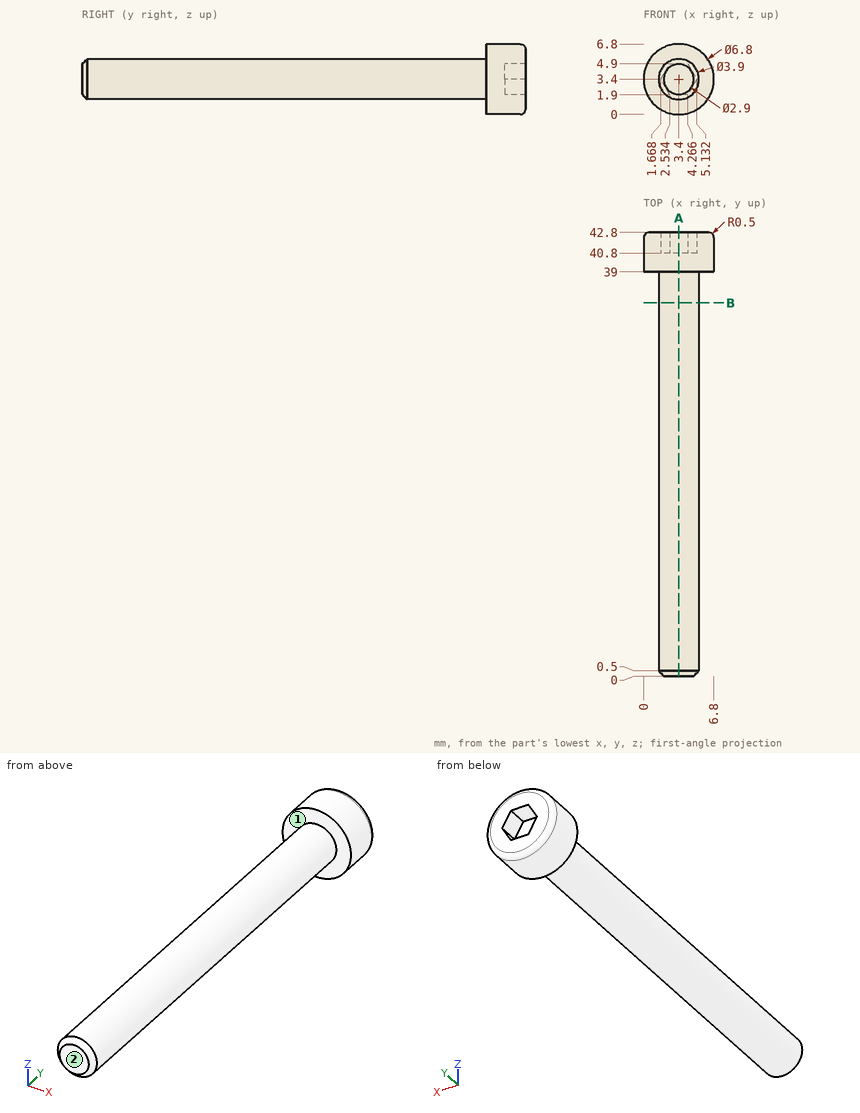
Print and shaded views of the part. All mm, measured from the part's lowest x, y and z. A direction names the side the tool comes from. Give positions to 0.01 mm unless a question says otherwise; leave off trailing zeros. Write each loop counter-clockwise with the first axis right and the second up, starting at its lowest first coordinate (ties: lowest second). Pieces come first, ordered by that corner, then holes. Notation, with made-up numbers: (29.5, 87.25) -> (70.5, 87.25) arc R33 cw to (70.5, 126.25) -> close; hole circle Ø10 at (47, 54). An arc over 180 degrees is marked (long way). Write each question's results on one line, items separated by ' | '.
1. Drop flat-ended pins along their axis: P1, Ø2, axis at y = 26.5, z = 4.5, coming from the -X side; P2, Ø1, axis at x = 4, y = 31, coming from the +Z side; P3, Ø3.5, axis at x = 2.5, z = 3.5, coming from the +Y side. Give the stop position or say it passes through.
Geometry check:
P1: x = 1.45 | P2: z = 5.35 | P3: y = 42.8
2. Which spindle directions (+Z, -Z, +X, -X, +Y, -Y) get a long thin tool onto all of the face, cutting with end or side? Do the marked faces 1 and 2. Say none if no direction does.
Geometry check:
face 1: -Y | face 2: +Z, -Z, +X, -X, -Y
3. Cut at B-B, the plane y = 36. Write the cut outline in (x, z), then the cut area to 3 significant figures.
Geometry check:
outline: circle Ø3.9 at (3.4, 3.4) | area: 11.9 mm²
4. Wall check: probe 1 along Y at (x, z) = (2, 6); probe 2 along Z at (x, y) = (3.25, 7.5). Give the ranges that are in metal, low to high. Write a range as [from, to].
Geometry check:
probe 1: [39, 42.8] | probe 2: [1.46, 5.34]
5. Cut at A-A, the plane x = 3.4. Write the cut outline in (y, z), then the cut area to 3 significant figures.
Geometry check:
outline: (0, 1.95) -> (0.5, 1.45) -> (39, 1.45) -> (39, 0) -> (42.3, 0) arc R0.5 ccw to (42.8, 0.5) -> (42.8, 1.9) -> (40.8, 1.9) -> (40.8, 4.9) -> (42.8, 4.9) -> (42.8, 6.3) arc R0.5 ccw to (42.3, 6.8) -> (39, 6.8) -> (39, 5.35) -> (0.5, 5.35) -> (0, 4.85) -> close | area: 172 mm²
